Geometry check sheet. Reference: drawing and pictorial views, mm from the part's lowest x, y, z. A direction names the side the tool comes from. Give positions to 0.01 mm unless a question says otherwise; leave off trailing zeros. Write each loop counter-clockwise with the first axis right and the second up, starting at its lowest first coordinate (ties: lowest second). Pieces come first, ordered by that corner, then holes. Notation, with made-up numbers: M 19.25,58.25 L 54.25,58.25 A9 ccw 54.25,74.25 Z; hole C 63,86.25 d4. An arc over 180 degrees is marked long. Write each question's results on one line, items separated by ' | '. Start each with the question number.
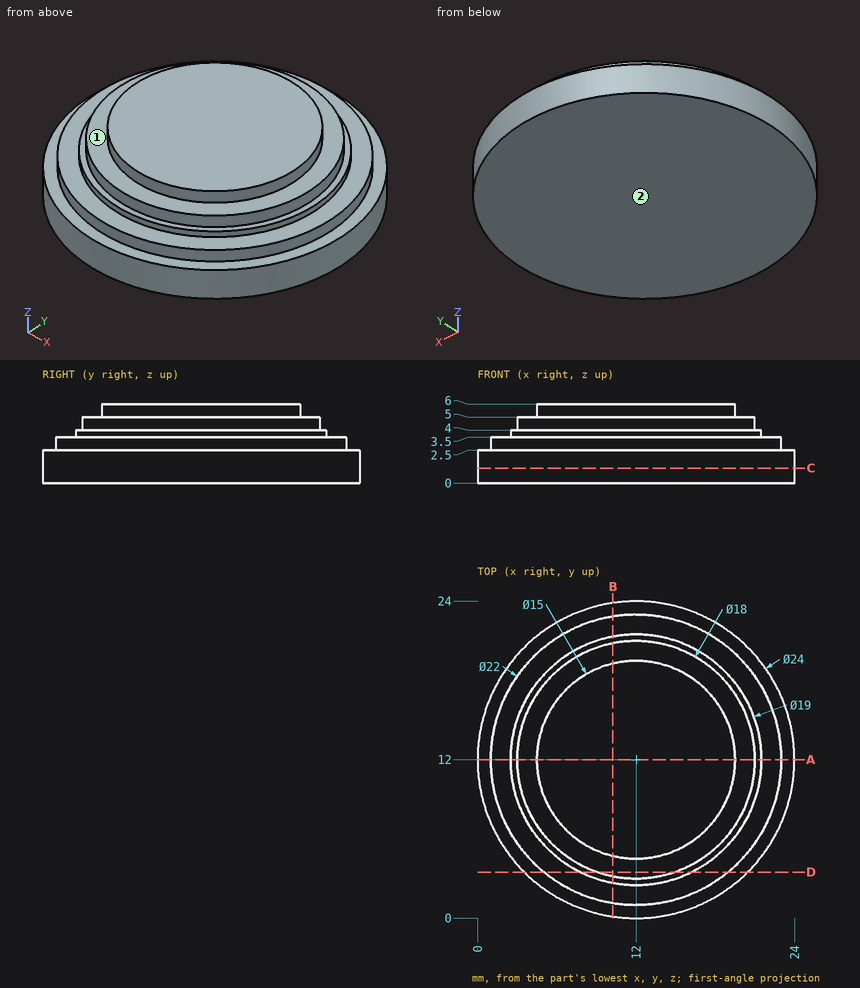
Q1. Depth check by flat-ended pin: pin 1 Ø1.5 at (x, y) = (17, 2.5) entering from -Z; pin 2 Ø1.5 at (x, z) = (20, 5) entering from +Y; pin 3 Ø2 at (y, z) = (21.5, 1) entering from -X. Enter the tip coordinate at first touch or a pass-through.
Q2. Tool access check on the marked faces 1 and 2. Record the directions out of +Z, -Z, +X, -X, +Y, -Y that give a thin tool (end or side, any length) a straight path to the whole face; none if there is none.
Q3. Scan lines: L1, parallel to Z at x = 19.5, y = 2.75; L2, parallel to Z at x = 16.5, y = 21.75; L3, parallel to Y at x = 5.75, z = 3.1. Record each from-to range of solid material in increasing order.
Q4. Section check D-D on y = 3.5. Record the boundary of the cut face in (x, z), plus the area to 3 significant figures.
Q5. Section check A-A on y = 12. Record the boundary of the cut face in (x, z).
Q6. Section check C-C on z = 1.15. Record the boundary of the cut face in (x, y), plus the area to 3 significant figures.
Q7. Section check B-B on x = 10.25. Record the boundary of the cut face in (y, z), plus the area to 3 significant figures.
Check result:
1) pin 1: z = 0 | pin 2: y = 17.33 | pin 3: x = 3.53
2) face 1: +Z | face 2: -Z, +X, -X, +Y, -Y
3) L1: 0 to 2.5 | L2: 0 to 3.5 | L3: 2.95 to 21.05
4) outline: M 3.53,0 L 20.47,0 L 20.47,2.5 L 18.98,2.5 L 18.98,3.5 L 16.24,3.5 L 16.24,4 L 14.96,4 L 14.96,5 L 9.04,5 L 9.04,4 L 7.76,4 L 7.76,3.5 L 5.02,3.5 L 5.02,2.5 L 3.53,2.5 Z | area: 66.5 mm^2
5) outline: M 0,0 L 24,0 L 24,2.5 L 23,2.5 L 23,3.5 L 21.5,3.5 L 21.5,4 L 21,4 L 21,5 L 19.5,5 L 19.5,6 L 4.5,6 L 4.5,5 L 3,5 L 3,4 L 2.5,4 L 2.5,3.5 L 1,3.5 L 1,2.5 L 0,2.5 Z
6) outline: C 12,12 d24 | area: 452 mm^2
7) outline: M 0.13,0 L 23.87,0 L 23.87,2.5 L 22.86,2.5 L 22.86,3.5 L 21.34,3.5 L 21.34,4 L 20.83,4 L 20.83,5 L 19.29,5 L 19.29,6 L 4.71,6 L 4.71,5 L 3.17,5 L 3.17,4 L 2.66,4 L 2.66,3.5 L 1.14,3.5 L 1.14,2.5 L 0.13,2.5 Z | area: 123 mm^2
